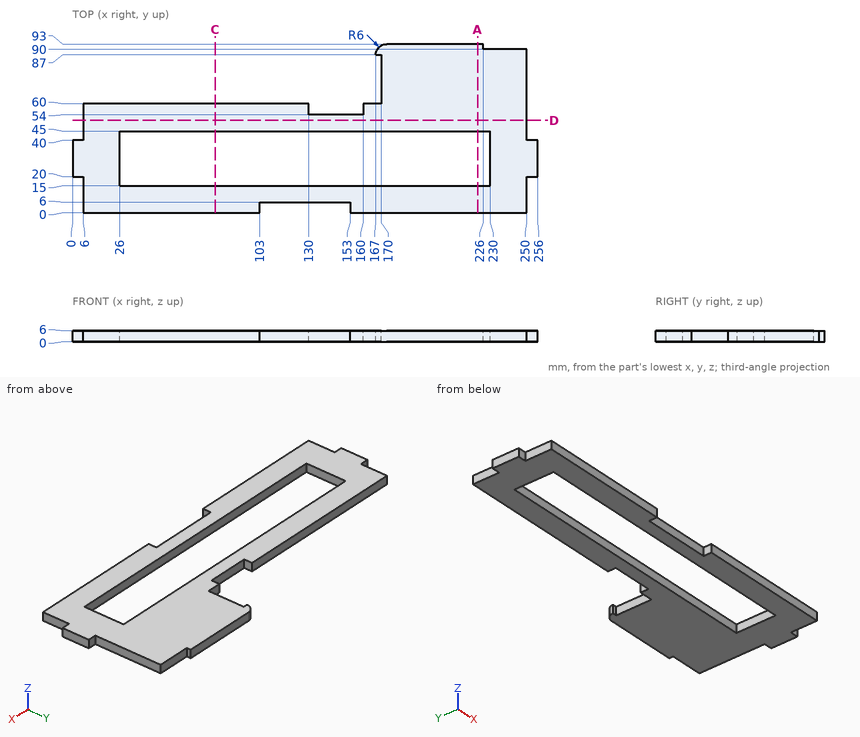
Study the drawing (mm; zero at the part's minimum x, y, z) and answer. Give positions to 0.01 mm unless a question says otherwise; leave off trailing zeros. Loops run counter-clockwise (first coordinate to the right, second up) from the corner with the lowest first, then second, coordinate; pieces in that order, holes last. Notation, with made-up numbers: (-4.75, 60) - (34.25, 60) arc R22 cw to (34.25, 79) - close; hole circle Ø6 at (59.25, -10). An arc over 180 degrees is marked (long way). Answer in a Markdown table with one row per item. Add a question column.
Q1. The part is cut by section A-A (x = 223). Determine the outline of the cut face in (y, z).
Q2. Each of these flat-tipped pins is pushed along its axis until it touches: P1, Ø1.8, axis at y = 11, z = 2.5, coming from the +X side; P2, Ø1.8, axis at x = 140.5, z = 2.5, coming from the -Y side; P3, Ø3, axis at x = 141, z = 4, coming from the +Y side. Where does it stop, or does it pass through?
Q3. The part is cut by section C-C (x = 78.5). Determine the outline of the cut face in (y, z), and give its area (3 significant figures).
Q4. Consider line 1 along X through (y, z) = (38, 1.8); line 2 along X through (y, z) = (19, 2.8); line 3 along Y through (x, z) = (128, 0.65). Determine where each line is inside the solid, lowest interval first.
Q5. The part is cut by section D-D (y = 51). Determine the outline of the cut face in (x, z).
Solution:
| question | item | result |
|---|---|---|
| 1 | outline | (0, 0) - (15, 0) - (15, 6) - (0, 6) - close; (45, 0) - (93, 0) - (93, 6) - (45, 6) - close |
| 2 | P1 | stops at x = 250 |
| 2 | P2 | stops at y = 6 |
| 2 | P3 | stops at y = 54 |
| 3 | outline | (0, 0) - (15, 0) - (15, 6) - (0, 6) - close; (45, 0) - (60, 0) - (60, 6) - (45, 6) - close |
| 3 | area | 180 mm² |
| 4 | line 1 | x = 0 to 26, 230 to 256 |
| 4 | line 2 | x = 6 to 26, 230 to 250 |
| 4 | line 3 | y = 6 to 15, 45 to 60 |
| 5 | outline | (6, 0) - (250, 0) - (250, 6) - (6, 6) - close |
